```python
from build123d import *

# Parameters (mm, degrees)
SKETCH_1_R          = 5
EXTRUDE_1_DEPTH     = 602
CHAMFER_1_SIZE      = 0.5
CUT_EXTRUDE_2_DEPTH = 10


with BuildPart() as part:
    # 草图1 → 拉伸1 (new body)
    with BuildSketch(Plane.XY):
        Circle(SKETCH_1_R)
    extrude(amount=EXTRUDE_1_DEPTH)

    # 倒角1
    chamfer_1_edges = [part.edges().sort_by_distance(p)[0] for p in [
        (-5, 0, 0),
        (-5, 0, 602),
    ]]
    chamfer(chamfer_1_edges, length=CHAMFER_1_SIZE)

    # 草图2 → 拉伸2 (cut)
    with BuildSketch(Plane(origin=(0, 2.5, 0), x_dir=(-1, 0, 0), z_dir=(0, 1, 0))):
        with BuildLine():
            Line((2, 472), (2, 447))
            ThreePointArc((2, 447), (0, 445), (-2, 447))
            Line((-2, 447), (-2, 472))
            ThreePointArc((-2, 472), (0, 474), (2, 472))
        make_face()
    extrude(amount=CUT_EXTRUDE_2_DEPTH, mode=Mode.SUBTRACT)


solid = part.part
```
The listing builds one solid part. Answer for the finished solid, in the listing's coordinates (mm). Coordinates: 2 decimals unless noted, no trailing zeros. Write each loop counter-clockwise with the first axis right and the second up, starting at its lowest first coordinate (ties: lowest second). Pieces come first, ordered by that corner, then holes. Notation, with made-up numbers: (34.25, 7) - (44.25, 7) arc R10 cw to (44.25, 26) - close; hole circle Ø3 at (21, 33.5). An arc over 180 degrees is marked (long way). One line per item, written item: value.
1) Find section A-A (z = 494). Give the vertices of the cut face in (x, y).
Geometry check:
outline: circle Ø10 at (0, 0)
2) Each of these flat-tipped pins is pushed along its axis until it touches: pin 1 Ø5 at (x, z) = (4, 160) entering from +Y; pin 2 Ø1 at (y, z) = (3.5, 463) entering from +X; pin 3 Ø2.5 at (y, z) = (3.5, 454) entering from -X. Where does it stop, or does it pass through?
Geometry check:
pin 1: stops at y = 4.77
pin 2: stops at x = 4
pin 3: stops at x = -4.47
3) Consider line 1 along X through (y, z) = (1, 61); line 2 along Y through (x, z) = (0.5, 397); line 3 along Z through (x, y) = (0.75, 4.75). Determine where each line is inside the solid, lowest interval first. Write a range as from..to.
Geometry check:
line 1: x = -4.9..4.9
line 2: y = -4.97..4.97
line 3: z = 0.31..445.15, 473.85..601.69
